Work out the finished part from the listing and answer in its coordinate system (mm). Face numbers are marked on the shaded views. A direction names the side the tool comes from. Give positions to 0.01 mm unless a question says otherwise; leave off trailing zeros. Loops run counter-clockwise (first coordinate to the right, second up) from the corner with the lowest first, then second, coordinate; pieces in that order, holes last. Notation, with made-up numbers: (64.5, 21) -> (108.5, 21) arc R18 ccw to (108.5, 44) -> close; hole circle Ø11 at (56.5, -6). An arc over 180 degrees is marked (long way). Answer as CSV lines item,"result". Start each with the question number.
1. A tool of negligible diameter and unlimited length cuts with its end or side. For the marked faces 4, 5, 6 and 7, from which of +Z, -Z, +X, -X, +Y, -Y can it reach the whole face along a straight path? Write none if from no direction.
2. Find section A-A, the plane z = -42.5. Give the vertices of the cut face in (x, y), and give its area (3 significant figures).
3. Find section B-B, the plane y = 15. Give the vertices of the cut face in (x, z).
4. Find the intervals of material crossed by line 1 along Z through (x, y) = (-8, 3); line 2 along Z through (x, y) = (10, 3.5); line 3 along X through (y, z) = (13.5, -56.5), in increasing order.
5. Find section D-D, the plane z = -18. Give the vertices of the cut face in (x, y), and give its area (3 significant figures).
6. Find section C-C, the plane x = -2.5. Give the vertices of the cut face in (y, z).
7. Flat-ended cylindrical pins translate along their axes: pin 1 Ø3 at (x, z) = (21, -58) entering from -Y; pin 2 Ø4 at (x, y) = (-30.5, 28) entering from +Z; pin 3 Ø22.5 at (x, z) = (-15, -45) entering from -Y. Find the tip coordinate at first contact, or state that the pin passes through.
8. Determine the mould class of the marked faces 1, 2 and 3 for opening direction Z: +Z half, -Z half, draft (parallel to the pull), parting line (faces both ways), or undercut.
from build123d import *

# Parameters (mm, degrees)
SKETCH1_W           = 130
SKETCH1_H           = 80
BOSS_EXTRUDE1_DEPTH = 45
BOSS_EXTRUDE3_DEPTH = 80
CUT_EXTRUDE1_DEPTH  = 20
FILLET2_R           = 2.5
SHELL2_START        = -76
SHELL2_OUTLINE_W    = 122
SHELL2_OUTLINE_H    = 41
SHELL2_DEPTH        = 72
SHELL2_2_DEPTH      = 52
SKETCH9_W           = 130
SKETCH9_H           = 80
BOSS_EXTRUDE7_DEPTH = 20
SKETCH9_3_W         = 126
SKETCH9_3_H         = 76
CUT_EXTRUDE3_DEPTH  = 15
SKETCH10_W          = 25
SKETCH10_H          = 15
CUT_EXTRUDE4_DEPTH  = 15


# Read off the part's stored shape, not the designer's step: Shell2
with BuildPart() as part:
    # Sketch1 → Boss-Extrude1 (new body)
    with BuildSketch(Plane(origin=(0, 0, 0), x_dir=(1, 0, 0), z_dir=(0, 1, 0))):
        with Locations((65, 40)):
            Rectangle(SKETCH1_W, SKETCH1_H)
    extrude(amount=BOSS_EXTRUDE1_DEPTH)

    # Sketch3 → Boss-Extrude3 (add)
    with BuildSketch(Plane.XY):
        Polygon((0, 0), (0, 45), (-22.202683057, 45), (-46.951420398, 20.251262658), (-46.951420398, 0), align=None)
    extrude(amount=-BOSS_EXTRUDE3_DEPTH)

    # Sketch3<4> → Cut-Extrude1 (cut)
    with BuildSketch(Plane.XY):
        Polygon((0, 0), (0, 45), (-22.202683057, 45), (-46.951420398, 20.251262658), (-46.951420398, 0), align=None)
    extrude(amount=-CUT_EXTRUDE1_DEPTH, mode=Mode.SUBTRACT)

    # Fillet2
    fillet2_edges = [part.edges().sort_by_distance(p)[0] for p in [
        (-34.577051727, 32.625631329, -80),
        (-22.202683057, 45, -50),
        (-46.951420398, 20.251262658, -50),
        (-46.951420398, 10.125631329, -80),
        (-46.951420398, 10.125631329, -20),
        (-34.577051727, 32.625631329, -20),
    ]]
    fillet(fillet2_edges, radius=FILLET2_R)

    # Shell2 outline → Shell2 (cut)
    with BuildSketch(Plane.XY.offset(SHELL2_START)):
        with Locations((65, 20.5)):
            Rectangle(SHELL2_OUTLINE_W, SHELL2_OUTLINE_H)
    extrude(amount=SHELL2_DEPTH, mode=Mode.SUBTRACT)

    # Shell2 2 outline → Shell2 2 (cut)
    with BuildSketch(Plane.XY.offset(SHELL2_START)):
        Polygon((-20.545828807, 41), (-42.951420398, 18.594408409), (-42.951420398, 0), (4, 0), (4, 41), align=None)
    extrude(amount=SHELL2_2_DEPTH, mode=Mode.SUBTRACT)

    # Sketch9 → Boss-Extrude7 (add)
    with BuildSketch(Plane(origin=(0, 45, 0), x_dir=(1, 0, 0), z_dir=(0, 1, 0))):
        with Locations((65, 40)):
            Rectangle(SKETCH9_W, SKETCH9_H)
    extrude(amount=-BOSS_EXTRUDE7_DEPTH)

    # Sketch9<3> → Cut-Extrude3 (cut)
    with BuildSketch(Plane(origin=(0, 45, 0), x_dir=(1, 0, 0), z_dir=(0, 1, 0))):
        with Locations((65, 40)):
            Rectangle(SKETCH9_3_W, SKETCH9_3_H)
    extrude(amount=-CUT_EXTRUDE3_DEPTH, mode=Mode.SUBTRACT)

    # Sketch10 → Cut-Extrude4 (cut)
    with BuildSketch(Plane(origin=(-33.601341528, 33.601341528, 0), x_dir=(0, 0, 1), z_dir=(-0.7071067811865477, 0.7071067811865475, 0))):
        with Locations((-50, -1.379862597)):
            Rectangle(SKETCH10_W, SKETCH10_H)
    extrude(amount=-CUT_EXTRUDE4_DEPTH, mode=Mode.SUBTRACT)


solid = part.part
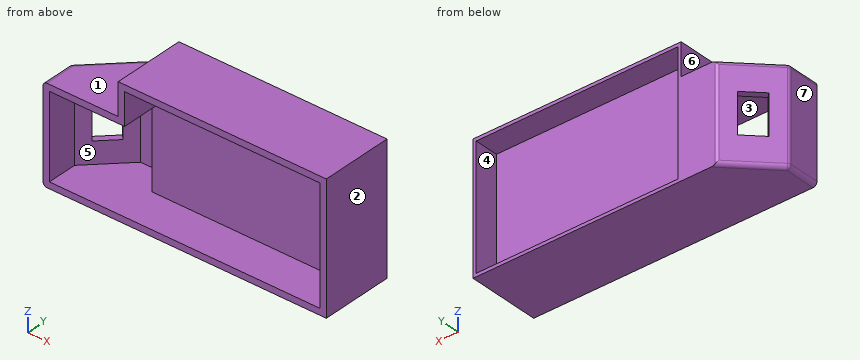
Resolved:
1,face 4,"+Y"
1,face 5,"-Y"
1,face 6,"+Z, -X, +Y, -Y"
1,face 7,"+Z, -Z, -X, +Y, -Y"
2,outline,"(-46.95, 0) -> (-42.95, 0) -> (-42.95, 18.59) -> (-37.05, 24.49) -> (-39.88, 27.32) -> (-46.22, 20.98) arc R2.5 ccw to (-46.95, 19.22) -> close; (-29.27, 37.93) -> (-26.45, 35.1) -> (-20.55, 41) -> (0, 41) -> (0, 25) -> (126, 25) -> (126, 0) -> (130, 0) -> (130, 45) -> (128, 45) -> (128, 30) -> (2, 30) -> (2, 45) -> (-21.17, 45) arc R2.5 ccw to (-22.93, 44.27) -> close"
2,area,"1,050 mm^2"
3,outline,"(-46.95, -77.5) arc R2.5 ccw to (-44.45, -80) -> (130, -80) -> (130, 0) -> (0, 0) -> (0, -20) -> (-44.45, -20) arc R2.5 ccw to (-46.95, -22.5) -> close; hole (-42.95, -76) -> (126, -76) -> (126, -4) -> (4, -4) -> (4, -24) -> (-42.95, -24) -> close"
4,line 1,"z = -80 to -76, -24 to -20"
4,line 2,"z = -80 to -76, -4 to 0"
4,line 3,"x = -46.95 to -42.95, 126 to 130"
5,outline,"(0, 0) -> (4, 0) -> (4, 25) -> (126, 25) -> (126, 0) -> (130, 0) -> (130, 45) -> (128, 45) -> (128, 30) -> (2, 30) -> (2, 45) -> (0, 45) -> close"
5,area,"910 mm^2"
6,outline,"(0, -80) -> (45, -80) -> (45, -20) -> (0, -20) -> (0, -24) -> (41, -24) -> (41, -76) -> (0, -76) -> close"
7,pin 1,"stops at y = 25"
7,pin 2,"stops at z = -20"
7,pin 3,"stops at y = 35.3"
8,face 1,"+Z half"
8,face 2,"draft"
8,face 3,"undercut"
